Part model, mm, in its own coordinate system. Face numbers are marked on the shaded views. A direction names the side the tool comes from. Give positions to 0.01 mm unless a question says otherwise; leave off trailing zeros. Write each loop counter-clockwise with the first axis right and the second up, starting at its lowest first coordinate (ties: lowest second). Pieces come first, ordered by that corner, then holes.
```python
from build123d import *

# Parameters (mm, degrees)
SKETCH2_R               = 2
SKETCH2_R_2             = 2.25
CUT_EXTRUDE1_DEPTH      = 5.5
CUT_EXTRUDE1_DEPTH_BACK = 5.5
SKETCH3_OUTSIDE_W       = 16.912
SKETCH3_OUTSIDE_H       = 42.61
CUT_EXTRUDE2_DEPTH      = 5.5
CUT_EXTRUDE2_DEPTH_BACK = 5.5


with BuildPart() as part:
    # Sketch1 → Revolve1 (revolve)
    with BuildSketch(Plane.XY, mode=Mode.PRIVATE) as revolve1_sk:
        with BuildLine():
            Line((0, 29), (0, -4.5))
            ThreePointArc((0, -4.5), (3.872392662, -2.292285993), (3.945169537, 2.1646333))
            ThreePointArc((3.945169537, 2.1646333), (3.770913113, 2.59367544), (3.7, 3.051292953))
            Line((3.7, 3.051292953), (3, 21.605833201))
            ThreePointArc((3, 21.605833201), (3.073295416, 22.222791768), (3.33238548, 22.787488528))
            ThreePointArc((3.33238548, 22.787488528), (3.524914601, 26.890760973), (0, 29))
        make_face()
    revolve(revolve1_sk.sketch.rotate(Axis((0, 0, 0), (0, 1, 0)), 90), axis=Axis((0, 0, 0), (0, 1, 0)))  # turned: the seam where the file's is

    # Sketch2 → Cut-Extrude1 (cut, two sides)
    with BuildSketch(Plane.XY) as cut_extrude1_sk:
        with Locations((0, 25)):
            Circle(SKETCH2_R)
        with Locations(Location((0, 0, 0), (0, 0, 74.166628888))):  # turned: the seam where the file's is
            Circle(SKETCH2_R_2)
    extrude(amount=CUT_EXTRUDE1_DEPTH, mode=Mode.SUBTRACT)
    extrude(cut_extrude1_sk.sketch, amount=-CUT_EXTRUDE1_DEPTH_BACK, mode=Mode.SUBTRACT)

    # Sketch3 outside → Cut-Extrude2 (cut, two sides)
    with BuildSketch(Plane(origin=(0, 0, 0), x_dir=(0, 0, -1), z_dir=(1, 0, 0))) as cut_extrude2_sk:
        with Locations((0, 12.25)):
            Rectangle(SKETCH3_OUTSIDE_W, SKETCH3_OUTSIDE_H)
        with BuildLine():
            Line((-2.5, 29), (2.5, 29))
            Line((2.5, 29), (2.5, 22))
            Line((2.5, 22), (2.25, 22))
            ThreePointArc((2.25, 22), (1.542893219, 21.707106781), (1.25, 21))
            Line((1.25, 21), (1.25, 5.468245837))
            ThreePointArc((1.25, 5.468245837), (1.459430585, 4.855873401), (2, 4.5))
            Line((2, 4.5), (2, -5))
            Line((2, -5), (-2, -5))
            Line((-2, -5), (-2, 4.5))
            ThreePointArc((-2, 4.5), (-1.459430585, 4.855873401), (-1.25, 5.468245837))
            Line((-1.25, 5.468245837), (-1.25, 21))
            ThreePointArc((-1.25, 21), (-1.542893219, 21.707106781), (-2.25, 22))
            Line((-2.25, 22), (-2.5, 22))
            Line((-2.5, 22), (-2.5, 29))
        make_face(mode=Mode.SUBTRACT)
    extrude(amount=CUT_EXTRUDE2_DEPTH, mode=Mode.SUBTRACT)
    extrude(cut_extrude2_sk.sketch, amount=-CUT_EXTRUDE2_DEPTH_BACK, mode=Mode.SUBTRACT)


solid = part.part
```
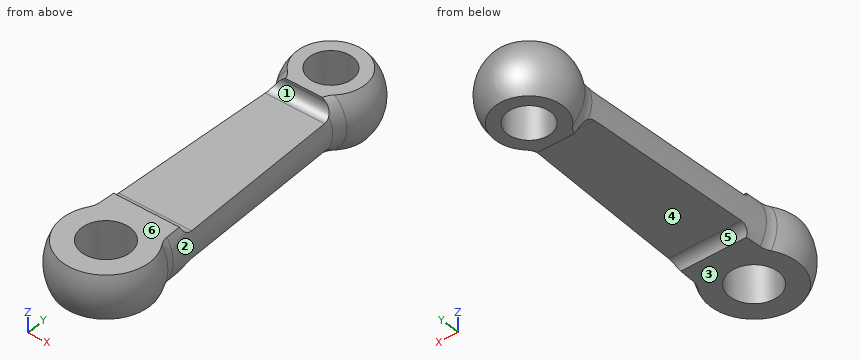
1) Pin check, flat tips, straight feed: pin 1 Ø3 at (x, y) = (0, 25) entering from +Z; pin 2 Ø1 at (y, z) = (13.5, 1.5) entering from -X; pin 3 Ø1.5 at (y, z) = (9, -1) entering from -X; pin 4 Ø3 at (x, z) = (-1, -2) entering from +Y. Stop position of each tip, or through.
Answers follow:
pin 1: passes through
pin 2: stops at x = -3.15
pin 3: stops at x = -3.47
pin 4: stops at y = 28.93
2) Wall check: L1, parallel to Y at x = 0, z = 1.4; L2, parallel to Y at x = -1.5, z = -0.7; L3, parallel to Y at x = -1.75, z = 0.9. Give the ranges that are in metal, low to high.
Answers follow:
L1: y = -4.28 to -2.25, 2.25 to 4.94, 21.53 to 23, 27 to 28.75
L2: y = -4.18 to -1.68, 1.68 to 23.68, 26.32 to 28.64
L3: y = -4.05 to -1.41, 1.41 to 24.03, 25.97 to 28.48
3) Saw through at A-A, the plane x = 0. Write the cut outline in (y, z), then the cut area to 3 significant figures.
Answers follow:
outline: (-4.03, -2) - (-2.25, -2) - (-2.25, 2) - (-4.03, 2) arc R4.5 ccw to start; (2.25, -2) - (4.5, -2) arc R1 cw to (5.47, -1.25) - (21, -1.25) arc R1 cw to (22, -2.25) - (22, -2.5) - (23, -2.5) - (23, 2.5) - (22, 2.5) - (22, 2.25) arc R1 cw to (21, 1.25) - (5.47, 1.25) arc R1 cw to (4.5, 2) - (2.25, 2) - close; (27, -2.5) - (28.12, -2.5) arc R4 ccw to (28.12, 2.5) - (27, 2.5) - close
area: 75.6 mm2
4) Two-plate mould, pull along Y, no slides. Class the marked faces 4, 5 and 6: +Y half, -Y half, draft (parallel to the pull), parting line (faces both ways), or undercut.
Answers follow:
face 4: undercut
face 5: undercut
face 6: draft
5) Saw through at B-B, the plane y = 25. Write the cut outline in (x, z).
Answers follow:
outline: (-3.12, -2.5) - (-2, -2.5) - (-2, 2.5) - (-3.12, 2.5) arc R4 ccw to start; (2, -2.5) - (3.12, -2.5) arc R4 ccw to (3.12, 2.5) - (2, 2.5) - close
6) 3-axis set-ups, long thin cutter, end or side, ignore diameter. For the marked faces 1, 2 and 3: which of +Z, -Z, +X, -X, +Y, -Y reach the whole face in a straight line?
Answers follow:
face 1: +Z, +X, -X
face 2: +X
face 3: -Z, +X, -X, -Y
7) Saw through at D-D, the plane x = -1.25. Write the cut outline in (y, z).
Answers follow:
outline: (-3.83, -2) - (-1.87, -2) - (-1.87, 2) - (-3.83, 2) arc R4.32 ccw to start; (1.87, -2) - (4.5, -2) arc R1 cw to (5.47, -1.25) - (21, -1.25) arc R1 cw to (22, -2.25) - (22, -2.5) - (23.44, -2.5) - (23.44, 2.5) - (22, 2.5) - (22, 2.25) arc R1 cw to (21, 1.25) - (5.47, 1.25) arc R1 cw to (4.5, 2) - (1.87, 2) - close; (26.56, -2.5) - (27.86, -2.5) arc R3.8 ccw to (27.86, 2.5) - (26.56, 2.5) - close
8) Saw through at C-C, the plane y = -0.5. Write the cut outline in (x, z).
Answers follow:
outline: (-4, -2) - (-2.19, -2) - (-2.19, 2) - (-4, 2) arc R4.47 ccw to start; (2.19, -2) - (4, -2) arc R4.47 ccw to (4, 2) - (2.19, 2) - close
